Study the drawing (mm; zero at the part's minimum x, y, z) and answer. A direction names the side the tool comes from. Coordinates: 2 decimals unless noted, no trailing zeros. Order: outer loops, then holes, each group sorted by start corner. A loop starts at its lowest first (then second) coordinate and runs counter-clockwise, first axis right, second up. Notation, with made-up numbers: M 57.5,-7 L 99.5,-7 A18 ccw 99.5,4 Z; hole C 46,4.25 d8. An arc over 180 degrees is marked long. Put each result on its own line as item: value.
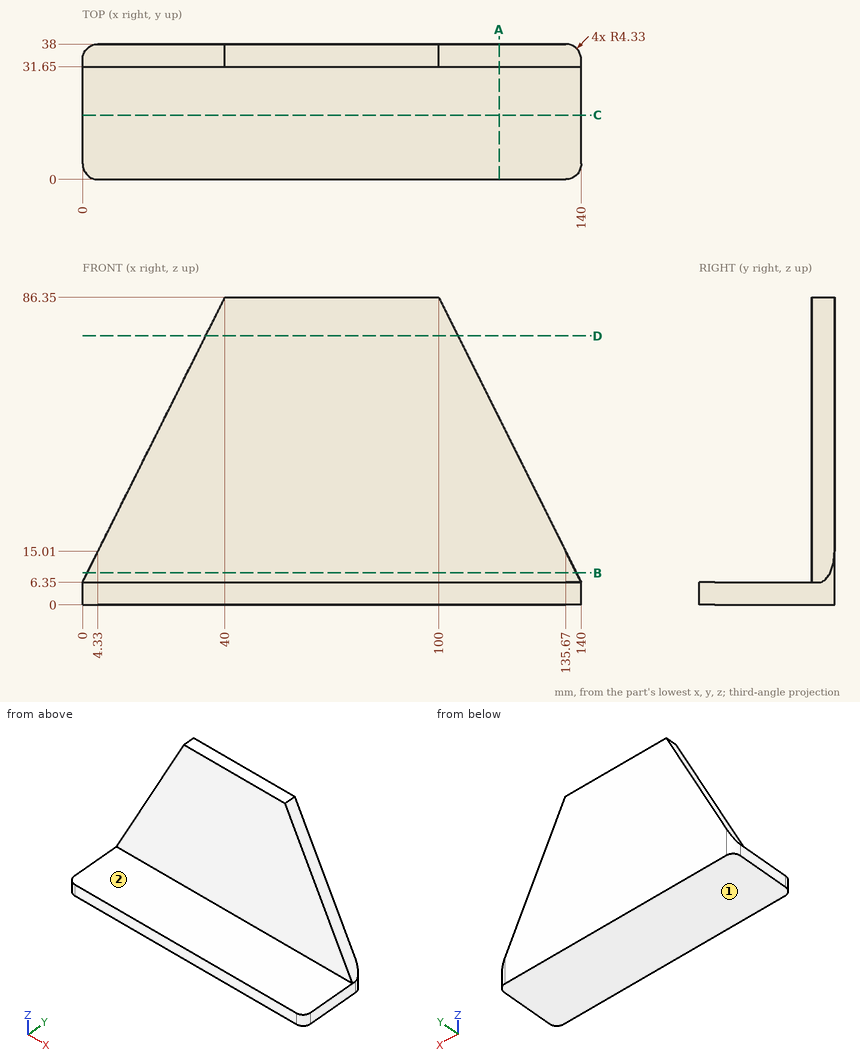
Q1. Find section B-B on z = 9. Write down the section's boundary in (x, y) (3 decimals), plus the area to 3 significant figures.
Answers below:
outline: M 1.325,31.65 L 138.675,31.65 L 138.675,36.788 A4.33 ccw 135.67,38 L 4.33,38 A4.33 ccw 1.325,36.788 Z
area: 870 mm^2
Q2. Given pin 1 (16 mm diameter, centred on x = 37.5, y = 13, fed in from +Z); pin 2 (3 mm diameter, centred on x = 95, y = 31, fed in from -Z); pin 3 (3 mm diameter, centred on x = 64, z = 53.5, fed in from -Y), each flat-ended and moving along its own axis, determine where each tip first touches the part or whether it passes through.
Answers below:
pin 1: stops at z = 6.35
pin 2: stops at z = 0
pin 3: stops at y = 31.65
Q3. Find section C-C on y = 18. Write down the section's boundary in (x, z), plus the area to 3 significant figures.
Answers below:
outline: M 0,0 L 140,0 L 140,6.35 L 0,6.35 Z
area: 889 mm^2
Q4. Consider line 1 along Y through (x, z) = (105.5, 48.5); line 2 along Z through (x, y) = (29, 9.5). Determine where each line is inside the solid, lowest interval first.
Answers below:
line 1: y = 31.65 to 38
line 2: z = 0 to 6.35
Q5. Find section A-A on x = 117. Write down the section's boundary in (y, z).
Answers below:
outline: M 0,0 L 38,0 L 38,52.35 L 31.65,52.35 L 31.65,6.35 L 0,6.35 Z
Q6. Find section D-D on z = 75.5. Write down the section's boundary in (x, y) (3 decimals).
Answers below:
outline: M 34.575,31.65 L 105.425,31.65 L 105.425,38 L 34.575,38 Z
Q7. A tool of negligible diameter and unlimited length cuts with its end or side. For the marked faces 1 and 2, from which of +Z, -Z, +X, -X, +Y, -Y can it reach the whole face along a straight path? Write none if from no direction.
Answers below:
face 1: -Z, +X, -X, +Y, -Y
face 2: +Z, +X, -X, -Y
